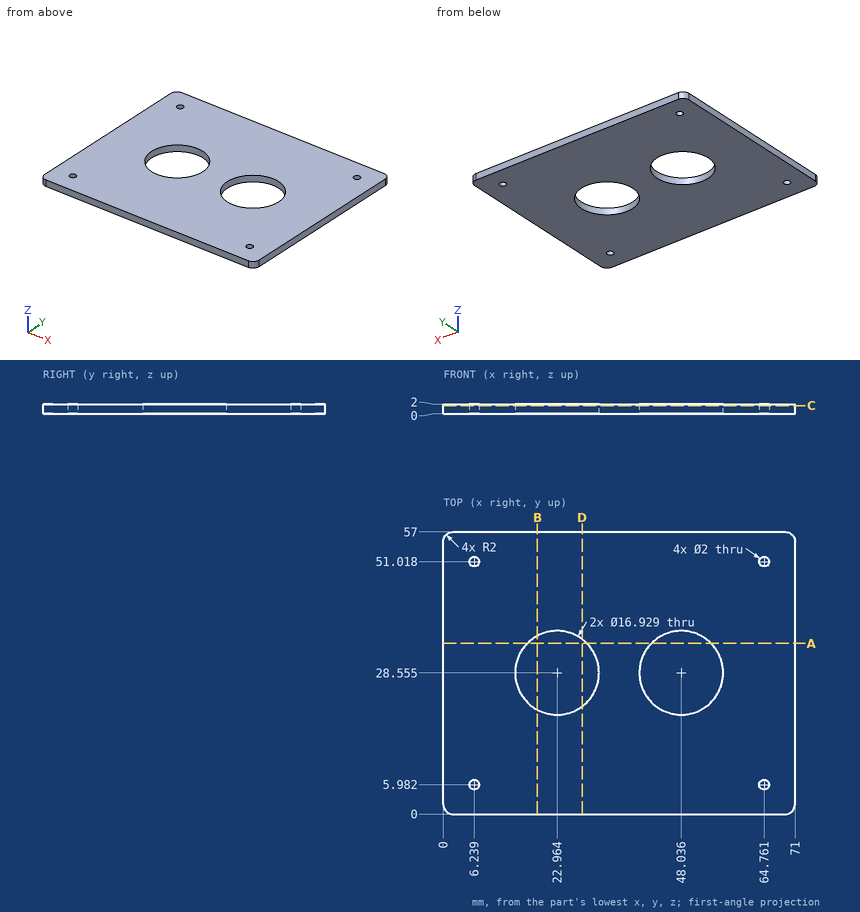
Part print with two shaded views. Sizes in mm from the minimum x, y, z corner. Round coordinates to 2 decimals unless told otherwise and drop trailing zeros. Write each loop counter-clockwise with the first axis right and the second up, starting at its lowest first coordinate (ties: lowest second). Pieces come first, ordered by that corner, then holes. Notation, with made-up numbers: M 48.5,64 L 55.5,64 A22 cw 55.5,100 Z; hole C 37,58 d10. An arc over 180 degrees is marked long. Use CSV: the item, a comma, the result in double quotes.
1. Saw through at B-B (x = 19). Give the cut face in (y, z).
Reply:
outline,"M 0,0 L 21.08,0 L 21.08,2 L 0,2 Z; M 36.03,0 L 57,0 L 57,2 L 36.03,2 Z"
2. Saw through at D-D (x = 28). Give the cut face in (y, z).
Reply:
outline,"M 0,0 L 21.75,0 L 21.75,2 L 0,2 Z; M 35.36,0 L 57,0 L 57,2 L 35.36,2 Z"
3. Saw through at C-C (z = 1.65). Give the cut face in (x, y) (1 decimal), plus the area to 3 significant figures.
Reply:
outline,"M 0,2 A2 ccw 2,0 L 69,0 A2 ccw 71,2 L 71,55 A2 ccw 69,57 L 2,57 A2 ccw 0,55 Z; hole C 6.2,6 d2; hole C 6.2,51 d2; hole C 23,28.6 d16.9; hole C 48,28.6 d16.9; hole C 64.8,6 d2; hole C 64.8,51 d2"
area,"3,580 mm²"
4. Wall check: probe 1 along X at (y, z) = (6, 1); probe 2 along X at (y, z) = (33.5, 0.3) (1 decimal); probe 3 along Y at (x, z) = (28, 1.1). Give the ranges that are in metal, low to high. Write a range as from..to.
Reply:
probe 1,"x = 0..5.24, 7.24..63.76, 65.76..71"
probe 2,"x = 0..16.1, 29.8..41.2, 54.9..71"
probe 3,"y = 0..21.75, 35.36..57"
5. Saw through at A-A (y = 34.5). Give the cut face in (x, z).
Reply:
outline,"M 0,0 L 16.94,0 L 16.94,2 L 0,2 Z; M 28.99,0 L 42.01,0 L 42.01,2 L 28.99,2 Z; M 54.06,0 L 71,0 L 71,2 L 54.06,2 Z"
6. Flat gauge pin, fed straight in: pin 1 (1.8 mm diameter, centred on x = 6.24, y = 5.98, fed in from +Z). Where does the tip first touch, or does it go through?
Reply:
pin 1,"passes through"
